Source: three-view drawing plus pictorial views. Frame: mm from the lowest corner of the part. Give positions to 0.01 mm unless a question says otherwise; leave off trailing zeros. Order: outer loops, then holes, each group sorted by start corner. A loop starts at its lowest first (then second) coordinate and runs counter-clockwise, first axis right, second up. Notation, with made-up numbers: (-26, 40.25) - (26, 40.25) arc R20 ccw to (26, 77.25) - close; hole circle Ø5 at (33, 83.5). An arc over 180 degrees is marked (long way). Use CSV: the item, a comma, the result in double quotes.
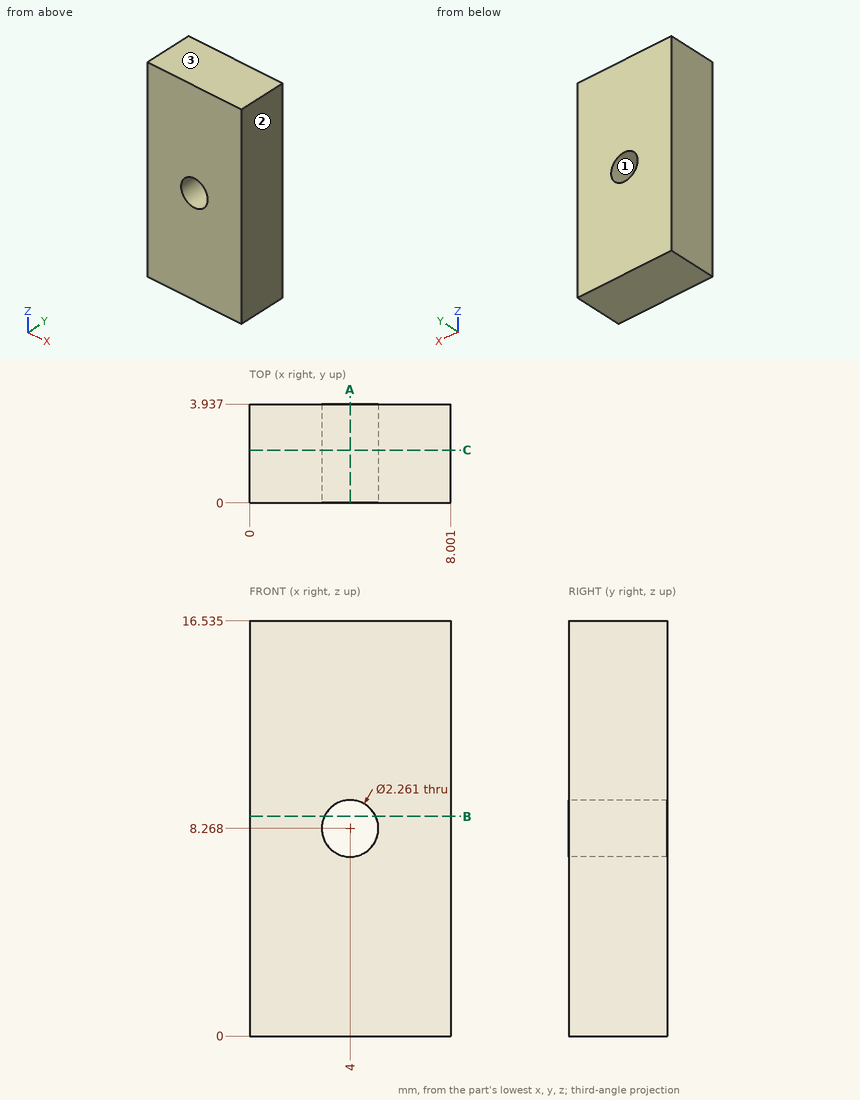
Item 1: Mould query, pull axis Z, two halves, no side actions, for the marked faces 1, 2 and 3. Classes: released by +Z, released by -Z, zero draft, split by the parting line, or undercut.
Filled in:
face 1,"undercut"
face 2,"zero draft"
face 3,"released by +Z"
Item 2: Section C-C on y = 2.1. Return the cut outline in (x, z) (1 decimal).
Filled in:
outline,"(0, 0) - (8, 0) - (8, 16.5) - (0, 16.5) - close; hole circle Ø2.3 at (4, 8.3)"
Item 3: Section B-B on z = 8.75. Return the cut outline in (x, y).
Filled in:
outline,"(0, 0) - (2.98, 0) - (2.98, 3.94) - (0, 3.94) - close; (5.02, 0) - (8, 0) - (8, 3.94) - (5.02, 3.94) - close"
Item 4: Material intervals for line 1 (Z direction, x = 3.25, y = 3.2) (1 decimal); line 2 (Z direction, x = 3, y = 0.4) (1 decimal); line 3 (X direction, y = 1.6, z = 8.75), sorted ascending. Write a range as from..to.
Filled in:
line 1,"z = 0..7.4, 9.1..16.5"
line 2,"z = 0..7.7, 8.8..16.5"
line 3,"x = 0..2.98, 5.02..8"
Item 5: First-contact query: pin 1 (2 mm diameter, centred on y = 3.5, z = 4.5, fed in from -X). Flat tip, straight axial feed; report the tip coordinate or a pass-through.
Filled in:
pin 1,"stops at x = 0"
Item 6: Section A-A on x = 4. Return the cut outline in (y, z) (1 decimal), then the cut area to 3 significant figures.
Filled in:
outline,"(0, 0) - (3.9, 0) - (3.9, 7.1) - (0, 7.1) - close; (0, 9.4) - (3.9, 9.4) - (3.9, 16.5) - (0, 16.5) - close"
area,"56.2 mm2"
